Autodesk Inventor part; units mm, degrees
ref_plane "YZ Plane" through (0, 0, 0) normal (1, 0, 0) x (0, 1, 0)
ref_plane "XZ Plane" through (0, 0, 0) normal (0, 1, 0) x (-1, 0, 0)
ref_plane "XY Plane" through (0, 0, 0) normal (0, 0, 1) x (1, 0, 0)
sketch "Sketch1" plane through (0, 0, 0) normal (1, 0, 0) x (0, 1, 0)
  line L0 (0, 0) -> (27, 0)
  line L1 (27, 0) -> (27, -55)
  line L2 (27, -55) -> (0, -55)
  line L3 (0, -55) -> (0, 0)
  dimension "d0" = 27
  dimension "d1" = 55
extrude "Extrusion1" add sketch "Sketch1" along normal blind 30
sketch "Sketch2" plane through (30, 0, 0) normal (1, 0, 0) x (0, 0, -1)
  line L0 (-2, 29) -> (57, 29)
  line L1 (57, 29) -> (57, -2)
  line L2 (57, -2) -> (-2, -2)
  line L3 (-2, -2) -> (-2, 29)
  line L4 (0, 27) -> (0, 0)
  line L5 (55, 27) -> (0, 27)
  line L6 (0, 0) -> (55, 0)
  line L7 (55, 0) -> (55, 27)
  dimension "d4" = 2
  dimension "d5" = 2
  dimension "d6" = 2
  dimension "d7" = 2
extrude "Extrusion2" add sketch "Sketch2" against normal blind 1
fillet "Fillet1" radius 2 4 edges at (29.5, 29, 2) (29.5, 29, -57) (29.5, -2, -57) (29.5, -2, 2)
sketch "Sketch3" plane through (30, 0, 0) normal (1, 0, 0) x (0, 0, -1)
  line L0 (6, 1) -> (18, 1)
  line L1 (18, 1) -> (18, 26)
  line L2 (18, 26) -> (6, 26)
  line L3 (1, 26) -> (1, 1)
  line L4 (0, 29) -> (55, 29)
  line L5 (55, -2) -> (0, -2)
  line L6 (1, 21) -> (6, 26)
  line L7 (1, 6) -> (6, 1)
  line L8 (-2, 0) -> (-2, 27)
  point P0 (0, 0)
  dimension "d11" = 17
  dimension "d12" = 25
  dimension "d13" = 31
  dimension "d14" = 3
  dimension "d15" = 3
  dimension "d16" = 5
  dimension "d17" = 5
  dimension "d18" = 5
  dimension "d19" = 5
extrude "Extrusion3" cut sketch "Sketch3" against normal blind 20
sketch "Sketch4" plane through (30, 0, 0) normal (1, 0, 0) x (0, 0, -1)
  line L0 (48.7705, 23.2756) -> (39.4061, 23.2756)
  line L1 (39.4061, 23.2756) -> (39.4061, 4.8716)
  line L2 (39.4061, 4.8716) -> (48.7705, 4.8716)
  line L3 (48.7705, 4.8716) -> (48.7705, 23.2756)
  point P0 (0, 0)
extrude "Extrusion4" add sketch "Sketch4" along normal blind 1
equation "\"d14\" = -0.5 * d12 + 0.5 * d13"
properties part number "power"
Here's how the part is built. I have some questions about the finished solid (model axes, mm). A direction names the side the tool comes from. Round coordinates to 2 decimals unless told otherwise and drop trailing zeros. Write each loop counter-clockwise with the first axis right and the second up, starting at its lowest first coordinate (ties: lowest second). Pieces come first, ordered by that corner, then holes.
1. For faces 1 (the flat face through (14, 27, -27)), 2 (the flat face through (20, 13, -18)), 3 (the flat face through (14, 0, -28)), 4 (the flat face through (14, 13, 0)), which set-ups out of +Z, -Z, +X, -X, +Y, -Y let a thin tool reach every point of the face, with its end or its side?
2. If we mould it in two halves opening along Z, with no side actions, what happens to faces 5 (the flat face through (14, 14, -55)), 6 (the cylindrical face through (29.49, 28.4, 1.43)), 7 (the flat face through (20, 26, -12))? For each: released by +Z, released by -Z, zero draft, split by the parting line, or undercut.
3. I need wall thicknesses on L1, parallel to Y at x = 24.5, z = -14.5; L2, parallel to Z at x = 23, y = 12; L3, parallel to Y at x = 16, z = -36.5. Which ranges of each line are inside material? Lowest first, please.
4. Will these pins go through, and if not, where does the flat tip stop? pin 1 Ø3 at (x, y) = (4, 2.5) entering from -Z; pin 2 Ø6 at (x, z) = (21.5, -13) entering from -Y; pin 3 Ø5 at (x, y) = (8.5, 13) entering from +Z.
5. Suppose I cut it at B-B (z = -8). List the corners of the cut face in (x, y) for me, and give its area (3 significant figures).
6. Suppose I cut it at A-A (x = 19.5). List the corners of the cut face in (y, z) for me.
7. Suppose I cut it at C-C (y = 24). List the corners of the cut face in (x, z) for me, and give its area (3 significant figures).
8. Suppose I cut it at D-D (z = -50). List the corners of the cut face in (x, y) for me.
Answer sheet:
1. face 1: +Z, -Z, -X, +Y
1. face 2: +X
1. face 3: +Z, -Z, -X, -Y
1. face 4: +Z, -X, +Y, -Y
2. face 5: released by -Z
2. face 6: released by +Z
2. face 7: undercut
3. L1: y = 0 to 1, 26 to 27
3. L2: z = -55 to -18, -1 to 0
3. L3: y = 0 to 27
4. pin 1: stops at z = -55
4. pin 2: stops at y = 0
4. pin 3: stops at z = 0
5. outline: (0, 0) - (29, 0) - (29, -2) - (30, -2) - (30, 1) - (10, 1) - (10, 26) - (30, 26) - (30, 29) - (29, 29) - (29, 27) - (0, 27) - close
5. area: 314 mm2
6. outline: (0, -55) - (27, -55) - (27, 0) - (0, 0) - close; hole (1, -18) - (26, -18) - (26, -6) - (21, -1) - (6, -1) - (1, -6) - close
7. outline: (0, -55) - (29, -55) - (29, -57) - (30, -57) - (30, -18) - (10, -18) - (10, -4) - (30, -4) - (30, 2) - (29, 2) - (29, 0) - (0, 0) - close
7. area: 1,370 mm2
8. outline: (0, 0) - (29, 0) - (29, -2) - (30, -2) - (30, 29) - (29, 29) - (29, 27) - (0, 27) - close
